```python
from build123d import *

# Parameters (mm, degrees)
F1_DEPTH = 25


with BuildPart() as f1:
    # F0 (on Top) → F1 (new body)
    with BuildSketch(Plane.XY):
        with BuildLine():
            Line((30, -48.34076), (30, 21.648188))
            ThreePointArc((30, 21.648188), (0, 51.648188), (-30, 21.648188))
            Line((-30, 21.648188), (-30, -48.34076))
            Line((-30, -48.34076), (-24, -48.34076))
            ThreePointArc((-24, -48.34076), (0, -24.34076), (24, -48.34076))
            Line((24, -48.34076), (30, -48.34076))
        make_face()
        with BuildLine():
            ThreePointArc((19.966583, 22.803858), (20, 21.648188), (19.966583, 20.492519))
            Line((19.966583, 20.492519), (19.966583, -20.821029))
            ThreePointArc((19.966583, -20.821029), (-0.020652, -14.340766), (-20, -20.845306))
            Line((-20, -20.845306), (-20, 21.648188))
            ThreePointArc((-20, 21.648188), (-0.578076, 41.639832), (19.966583, 22.803858))
        make_face(mode=Mode.SUBTRACT)
    extrude(amount=F1_DEPTH)


solid = f1.part
```
Here's how the part is built. I have some questions about the finished solid (model axes, mm). A direction names the side the tool comes from. Round coordinates to 2 decimals unless told otherwise and drop trailing zeros. Order: outer loops, then holes, each group sorted by start corner. A loop starts at its lowest first (then second) coordinate and runs counter-clockwise, first axis right, second up. Notation, with made-up numbers: (49.5, 29.25) -> (59.5, 29.25) arc R26 cw to (59.5, 50.25) -> close; hole circle Ø5 at (45, -27). An arc over 180 degrees is marked (long way). Use a Markdown table: item, result. Add a question column.
(1) For pin 1 Ø2 at (x, z) = (10, 21.5) entering from -Y; pin 2 Ø1.5 at (y, z) = (23, 14) entering from -X, each with a flat end and sliding along its axis, tell me the tip position at first contact or that it passes through.
(2) Suppose I cut it at B-B, the plane x = 0. Please give me the cut outline in (y, z), and give its area (3 significant figures).
(3) If we mould it in two halves opening along X, with no side actions, what happens to faces 1 (the face through (-20.4, 2.4, 0)), 2 (the face through (-1.009, 41.623, 12.325)), 3 (the face through (-30, -13, 12))? For each: released by +X, released by -X, zero draft, split by the parting line, or undercut.
(4) Suppose I cut it at C-C, the plane x = 12. Please give me the cut outline in (y, z), and give its area (3 significant figures).
(5) Suppose I cut it at A-A, the plane z = 22.25. Please give me the cut outline in (x, y), and give its area (3 significant figures).
(6) I need wall thicknesses on line 1 along X through (y, z) = (1.5, 14); line 2 along Y through (x, z) = (11.5, 2.25); line 3 along X through (y, z) = (-33, 20.5). Which ranges of each line are inside material? Lowest first, please.
(7) For faces 4 (the face through (20, 21.7, 12.3)), 5 (the face through (27, -48.341, 12)), which set-ups out of +Z, -Z, +X, -X, +Y, -Y let a thin tool reach every point of the face, with its end or its side?
Verdict:
| question | item | result |
|---|---|---|
| 1 | pin 1 | y = -27.01 |
| 1 | pin 2 | x = -29.99 |
| 2 | outline | (-24.34, 0) -> (-14.34, 0) -> (-14.34, 25) -> (-24.34, 25) -> close; (41.65, 0) -> (51.65, 0) -> (51.65, 25) -> (41.65, 25) -> close |
| 2 | area | 500 mm2 |
| 3 | face 1 | zero draft |
| 3 | face 2 | undercut |
| 3 | face 3 | released by -X |
| 4 | outline | (-27.56, 0) -> (-16.53, 0) -> (-16.53, 25) -> (-27.56, 25) -> close; (37.65, 0) -> (49.14, 0) -> (49.14, 25) -> (37.65, 25) -> close |
| 4 | area | 563 mm2 |
| 5 | outline | (-30, -48.34) -> (-24, -48.34) arc R24 cw to (24, -48.34) -> (30, -48.34) -> (30, 21.65) arc R30 ccw to (-30, 21.65) -> close; hole (-20, -20.85) arc R34 cw to (19.97, -20.82) -> (19.97, 20.49) arc R20 ccw to (19.97, 22.8) arc R20 ccw to (-20, 21.65) -> close |
| 5 | area | 2,560 mm2 |
| 6 | line 1 | -30 to -20, 19.97 to 30 |
| 6 | line 2 | -27.28 to -16.34, 38.01 to 49.36 |
| 6 | line 3 | -30 to -18.46, 18.46 to 30 |
| 7 | face 4 | +Z, -Z |
| 7 | face 5 | +Z, -Z, +X, -X, -Y |
